Read the model definition and answer for the solid it produces. Units are mm, in the model's axes. A direction names the side the tool comes from. Give positions to 0.01 mm unless a question says otherwise; leave off trailing zeros. Use a Markdown table: item, result. Add a question column.
Item 1: For faces 5 (the flat face through (-85, 0, 31)), 6 (the cylindrical face through (-85.49, -15.97, 32.71)), determine the directions among +Z, -Z, +X, -X, +Y, -Y from which every point of the face is accessible in a straight line to the end or side of a thin tool.
Item 2: The mould has two halves that part along X. Classify faces 1 (the flat face through (-59.749, -12, 30)), 2 (the conical face through (-87.858, -9.557, 32.864)), 3 (the flat face through (-85, -12, 55.548)), 4 (the conical face through (-85.916, -21.67, 34.152)): pulls with the +X half, pulls with the -X half, needs draft (parallel to the pull), parting line crosses it, or undercut.
Item 3: Consider probe 1 along Y at (x, z) = (-84, 35.5). Determine where the line is inside the solid, lowest interval first. Write a range as [from, to].
Item 4: Given P1, Ø2, axis at x = -91, z = 31.5, coming from the -Y side; P2, Ø5, axis at x = -87.59, z = 32.62, coming from the -Y side, each flat-ended and moving along its own axis, determine where each tip first touches the part or whether it passes through.
from build123d import *

# Parameters (mm, degrees)
F0_W           = 50
F0_H           = 50
F1_DEPTH       = 25
F3_D           = 4.2
F3_DEPTH       = 14.4
F3_CSINK_D     = 11.2
F3_CSINK_ANGLE = 90
F3_TIP         = 1.2618073


with BuildPart() as f1:
    # F0 (on Front) → F1 (new body)
    with BuildSketch(Plane.XZ):
        with Locations((-84.7486946732, 30.5484851895)):
            Rectangle(F0_W, F0_H)
    extrude(amount=F1_DEPTH)

    # F3
    with Locations(Plane.XZ.offset(25)):
        with Locations((-87.5890702009, 32.6180011034)):
            CounterSinkHole(F3_D / 2, F3_CSINK_D / 2, depth=F3_DEPTH, counter_sink_angle=F3_CSINK_ANGLE)
            with Locations((0, 0, -(F3_DEPTH + F3_TIP / 2))):  # 118° drill point
                Cone(0, F3_D / 2, F3_TIP, mode=Mode.SUBTRACT)


solid = f1.part
Filled in:
| question | item | result |
|---|---|---|
| 1 | face 5 | +Z, -Z, +X, -X, +Y |
| 1 | face 6 | -Y |
| 2 | face 1 | pulls with the +X half |
| 2 | face 2 | undercut |
| 2 | face 3 | needs draft |
| 2 | face 4 | undercut |
| 3 | probe 1 | [-24, 0] |
| 4 | P1 | y = -23.99 |
| 4 | P2 | y = -21.9 |
